Geometry: see drawing. Coordinates: mm, zero at the bounding-box minimum. A direction names the side the tool comes from. Round coordinates to 2 decimals unless told otherwise and drop trailing zeros. Loops run counter-clockwise (first coordinate to the right, second up) from the corner with the lowest first, then second, coordinate; pieces in that order, holes last. Notation, with made-up numbers: (45, 6.5) - (104, 6.5) arc R18 cw to (104, 31.5) - close; hole circle Ø4 at (-30, 0). An arc over 180 degrees is marked (long way). Use CSV: the item, a comma, the result in double quotes. Start each with the question number.
1. Access query for the marked faces 1 and 2. Directions: +Z, -Z, +X, -X, +Y, -Y. A direction counts if a zero-diameter tool reaches every point of the face in a straight line with its end or side. Return the directions, or none.
2. Cut plane D-D (x = 9). Return loops of the section in (y, z).
3. Pin query (flat end, axial travel): P1, Ø1.3, axis at y = 56.25, z = 40, coming from the +X side; P2, Ø4, axis at x = 21.5, y = 27, coming from the -Z side; P3, Ø1.5, axis at x = 32, y = 55.5, coming from the -Z side; P4, Ø8, axis at x = 20.5, y = 48.5, coming from the +Z side. Return the tip coordinate at first contact, or that it passes through.
4. Pull-direction query (Z, two-part tool) for the marked faces 3, 4 and 5; classes: +Z half, -Z half, draft (parallel to the pull), parting line (faces both ways), or undercut.
5. Cut plane B-B (z = 40). Return loops of the section in (x, y), and give its area (3 significant figures).
6. Cut plane A-A (y = 45). Return loops of the section in (x, z).
7. Material intervals for probe 1 along Y at (x, z) = (10, 40); probe 2 along Z at (x, y) = (8, 45); probe 3 along X at (y, z) = (16.5, 28.5), sorted ascending. Write a range as from..to.
8. Cut plane C-C (y = 62.5). Return loops of the section in (x, z), and give its area (3 significant figures).
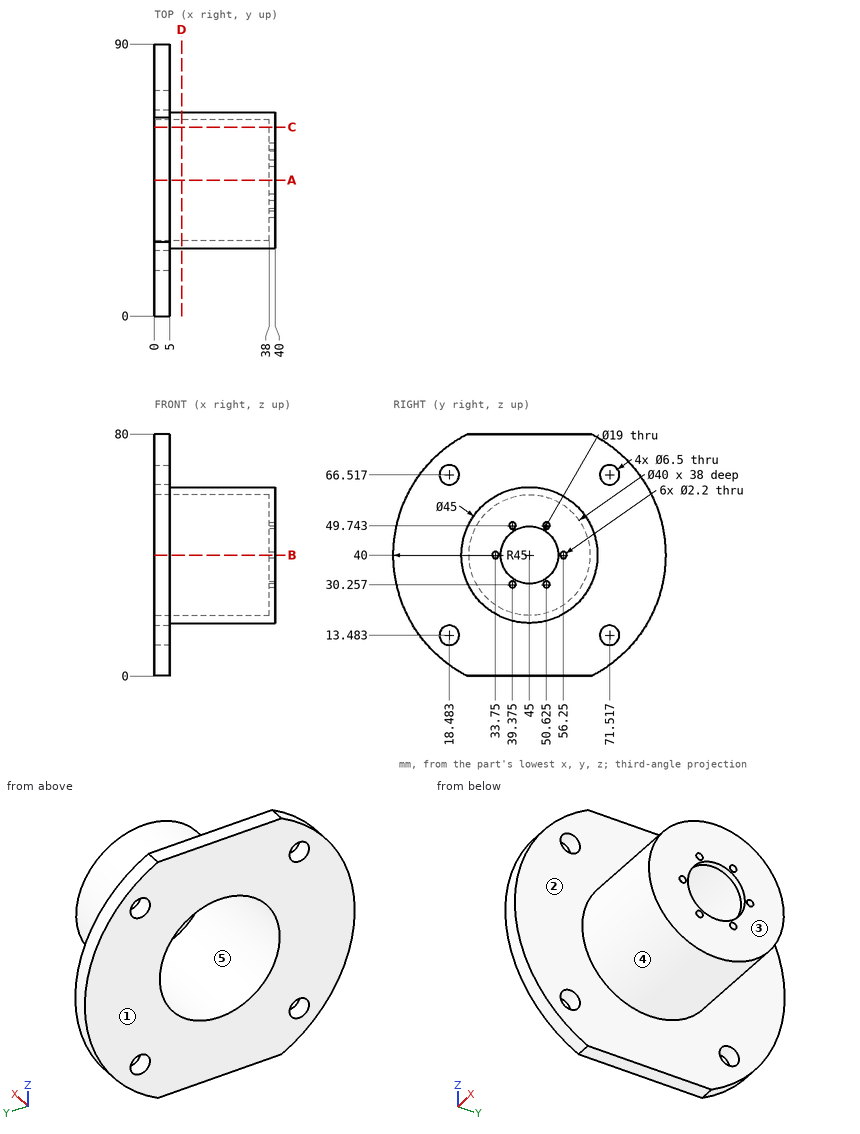
Established:
1,face 1,"+Z, -Z, -X, +Y, -Y"
1,face 2,"+X"
2,outline,"circle Ø45 at (45, 40); hole circle Ø40 at (45, 40)"
3,P1,"passes through"
3,P2,"stops at z = 24.18"
3,P3,"stops at z = 19.72"
3,P4,"stops at z = 62.5"
4,face 3,"draft"
4,face 4,"parting line"
4,face 5,"undercut"
5,outline,"(0, 0) - (5, 0) - (5, 22.5) - (40, 22.5) - (40, 32.65) - (38, 32.65) - (38, 25) - (0, 25) - close; (0, 65) - (38, 65) - (38, 57.35) - (40, 57.35) - (40, 67.5) - (5, 67.5) - (5, 90) - (0, 90) - close; (38, 34.85) - (40, 34.85) - (40, 35.5) - (38, 35.5) - close; (38, 54.5) - (40, 54.5) - (40, 55.15) - (38, 55.15) - close"
5,area,"458 mm2"
6,outline,"(0, 0) - (5, 0) - (5, 17.5) - (40, 17.5) - (40, 30.5) - (38, 30.5) - (38, 20) - (0, 20) - close; (0, 60) - (38, 60) - (38, 49.5) - (40, 49.5) - (40, 62.5) - (5, 62.5) - (5, 80) - (0, 80) - close"
7,probe 1,"y = 22.5..25, 65..67.5"
7,probe 2,"z = 17.5..20, 60..62.5"
7,probe 3,"x = 0..5"
8,outline,"(0, 0) - (5, 0) - (5, 25.86) - (40, 25.86) - (40, 54.14) - (5, 54.14) - (5, 80) - (0, 80) - (0, 49.68) - (38, 49.68) - (38, 30.32) - (0, 30.32) - close"
8,area,"654 mm2"
